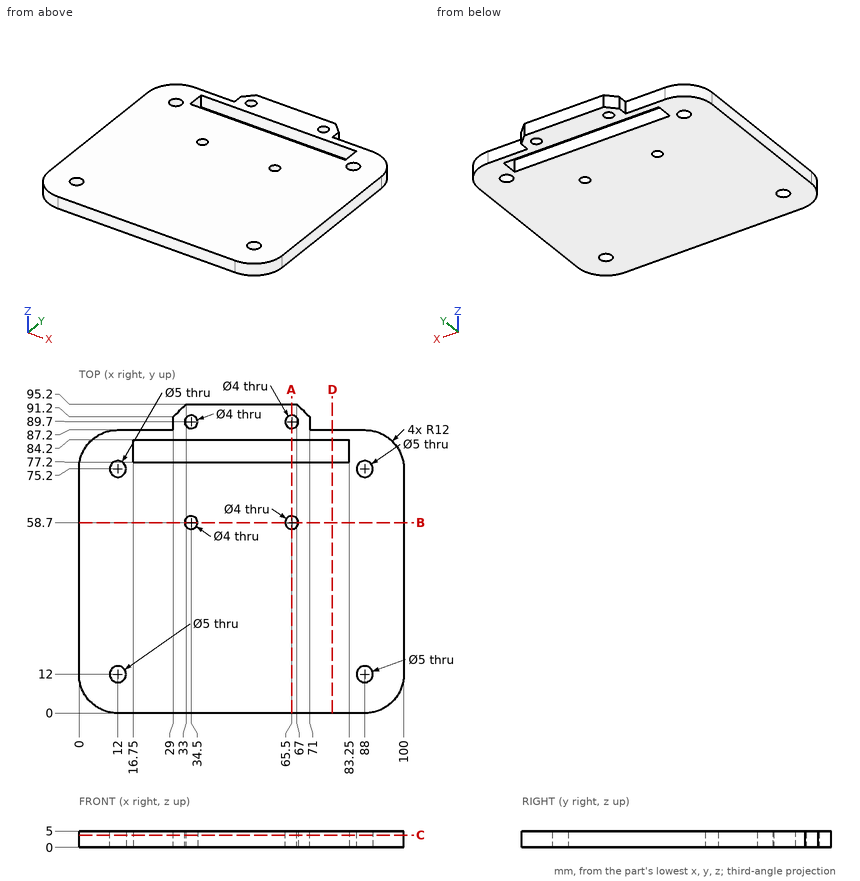
Print and shaded views of the part. All mm, measured from the part's lowest x, y and z. Give positions to 0.01 mm unless a question says otherwise; leave off trailing zeros. Loops run counter-clockwise (first coordinate to the right, second up) from the corner with the lowest first, then second, coordinate; pieces in that order, holes last. Notation, with made-up numbers: (8.5, 14.5) -> (46.5, 14.5) arc R24 ccw to (46.5, 37.5) -> close; hole circle Ø8 at (-13.5, 62). An arc over 180 degrees is marked (long way). Answer in a Markdown table with one row per item.
Item 1: Flat gauge pins, fed straight in: P1, Ø1.5, axis at y = 80.5, z = 2.5, coming from the -X side; P2, Ø6.5, axis at x = 65.5, y = 89.7, coming from the -Z side; P3, Ø2.5, axis at y = 81, z = 2.5, coming from the +X side; P4, Ø1.2, axis at y = 89.5, z = 2, coming from the -X side. Where does each tip first touch, or does it go through?
Findings below:
| item | result |
|---|---|
| P1 | stops at x = 0.9 |
| P2 | stops at z = 0 |
| P3 | stops at x = 99.1 |
| P4 | stops at x = 29 |
Item 2: Probe line 1 along Y through (x, z) = (34.5, 1.05); line 2 along Y through (x, z) = (88, 2.8); line 3 along Y through (x, z) = (20.5, 0.3). List the from-to ranges inside material, lowest first. Write a range as [from, to].
Findings below:
| item | result |
|---|---|
| line 1 | y = [0, 56.7], [60.7, 77.2], [84.2, 87.7], [91.7, 95.2] |
| line 2 | y = [0, 9.5], [14.5, 72.7], [77.7, 87.2] |
| line 3 | y = [0, 77.2], [84.2, 87.2] |
Item 3: Slice it at D-D on x = 78. Write the cut outline in (y, z).
Findings below:
| item | result |
|---|---|
| outline | (0, 0) -> (77.2, 0) -> (77.2, 5) -> (0, 5) -> close; (84.2, 0) -> (87.2, 0) -> (87.2, 5) -> (84.2, 5) -> close |
Item 4: Slice it at A-A on x = 65.5. Write the cut outline in (y, z).
Findings below:
| item | result |
|---|---|
| outline | (0, 0) -> (56.7, 0) -> (56.7, 5) -> (0, 5) -> close; (60.7, 0) -> (77.2, 0) -> (77.2, 5) -> (60.7, 5) -> close; (84.2, 0) -> (87.7, 0) -> (87.7, 5) -> (84.2, 5) -> close; (91.7, 0) -> (95.2, 0) -> (95.2, 5) -> (91.7, 5) -> close |
Item 5: Slice it at C-C on z = 3.8. Give the number of separate pieces and of enclosed holes in the cut face, plus the area to 3 significant figures.
Findings below:
| item | result |
|---|---|
| separate pieces | 1 |
| enclosed holes | 9 |
| area | 8,320 mm² |
Item 6: Slice it at B-B on y = 58.7. Write the cut outline in (x, z), plus the area to 3 significant figures.
Findings below:
| item | result |
|---|---|
| outline | (0, 0) -> (32.5, 0) -> (32.5, 5) -> (0, 5) -> close; (36.5, 0) -> (63.5, 0) -> (63.5, 5) -> (36.5, 5) -> close; (67.5, 0) -> (100, 0) -> (100, 5) -> (67.5, 5) -> close |
| area | 460 mm² |
